Part model, mm, in its own coordinate system. Round coordinates to 2 decimals unless told otherwise and drop trailing zeros. Loops run counter-clockwise (first coordinate to the right, second up) from the corner with the lowest first, then second, coordinate; pieces in that order, holes last. Notation, with made-up numbers: M -10,15 L 48,15 A19 ccw 48,48 Z; hole C 82,-23 d8. An arc over 180 degrees is marked long. Put each result on its own line as item: value. Start each with the question number.
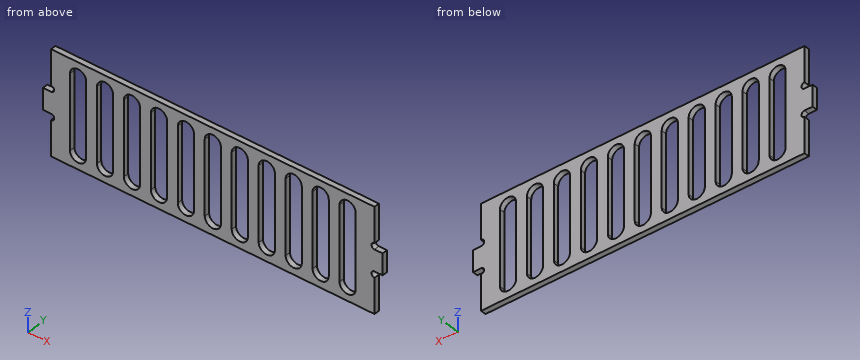
```python
from build123d import *

# Parameters (mm, degrees)
SKETCH_1_W                 = 120
SKETCH_1_H                 = 39
EXTRUDE_1_DEPTH            = 2
SKETCH_2_W                 = 8
SKETCH_2_H                 = 2
EXTRUDE_2_DEPTH            = 3
SKETCH_3_R                 = 1.15
CUT_EXTRUDE_1_DEPTH        = 66.979163378
CUT_EXTRUDE_2_DEPTH        = 66.979163378
PATTERN_LINEAR_1_COUNT     = 6
PATTERN_LINEAR_1_PITCH     = 10
PATTERN_LINEAR_1_COL_COUNT = 6
PATTERN_LINEAR_1_COL_PITCH = 10


with BuildPart() as part:
    # 草图1 → 凸台-拉伸1 (new body)
    with BuildSketch(Plane(origin=(0, 0, 0), x_dir=(1, 0, 0), z_dir=(0, 1, 0))):
        Rectangle(SKETCH_1_W, SKETCH_1_H)
    extrude(amount=EXTRUDE_1_DEPTH)

    # 草图2 → 凸台-拉伸2 (add)
    with BuildSketch(Plane.ZY.offset(60)):
        with Locations((0, 1)):
            Rectangle(SKETCH_2_W, SKETCH_2_H)
    extrude_2 = extrude(amount=EXTRUDE_2_DEPTH)

    # 草图3 → 切除-拉伸1 (cut, through all)
    with BuildSketch(Plane(origin=(0, 2, 0), x_dir=(1, 0, 0), z_dir=(0, 1, 0))):
        with Locations((-60, 5.15)):
            Circle(SKETCH_3_R)
        with Locations((-60, -5.15)):
            Circle(SKETCH_3_R)
    cut_extrude_1 = extrude(amount=-CUT_EXTRUDE_1_DEPTH, mode=Mode.SUBTRACT)

    # 镜向1: 凸台-拉伸2, 切除-拉伸1 across plane
    add(extrude_2.mirror(Plane(origin=(0, 0, 0), x_dir=(0, 0, 1), z_dir=(1, 0, 0))))
    add(cut_extrude_1.mirror(Plane(origin=(0, 0, 0), x_dir=(0, 0, 1), z_dir=(1, 0, 0))), mode=Mode.SUBTRACT)

    # 草图4 → 切除-拉伸2 (cut, through all)
    with BuildSketch(Plane(origin=(0, 2, 0), x_dir=(1, 0, 0), z_dir=(0, 1, 0))):
        with BuildLine():
            ThreePointArc((-3, -14), (0, -11), (3, -14))
            Line((3, -14), (3, 14))
            ThreePointArc((3, 14), (0, 11), (-3, 14))
            Line((-3, 14), (-3, -14))
        make_face()
        with BuildLine():
            ThreePointArc((-3, 14), (0, 11), (3, 14))
            Line((3, 14), (-3, 14))
        make_face()
        with BuildLine():
            Line((-3, 14), (3, 14))
            ThreePointArc((3, 14), (0, 17), (-3, 14))
        make_face()
        with BuildLine():
            ThreePointArc((-3, -14), (0, -17), (3, -14))
            Line((3, -14), (-3, -14))
        make_face()
        with BuildLine():
            Line((-3, -14), (3, -14))
            ThreePointArc((3, -14), (0, -11), (-3, -14))
        make_face()
    cut_extrude_2 = extrude(amount=-CUT_EXTRUDE_2_DEPTH, mode=Mode.SUBTRACT)

    # 阵列(线性)1: 切除-拉伸2 ×6
    with Locations(*[(-i * PATTERN_LINEAR_1_PITCH, 0, 0) for i in range(1, PATTERN_LINEAR_1_COUNT)]):
        add(cut_extrude_2, mode=Mode.SUBTRACT)

    # 阵列(线性)1 col: 切除-拉伸2 ×6
    with Locations(*[(i * PATTERN_LINEAR_1_COL_PITCH, 0, 0) for i in range(1, PATTERN_LINEAR_1_COL_COUNT)]):
        add(cut_extrude_2, mode=Mode.SUBTRACT)


solid = part.part
```
1. Wall check: L1, parallel to Z at x = -30, y = 1.4; L2, parallel to Z at x = 19, y = 0.5. Give the ranges that are in metal, low to high.
2. Cut at A-A, the plane x = -30. Give the cut face in (y, z), and give its area (3 significant figures).
3. Cut at B-B, the plane y = 1.3. Give the number of separate pieces and of enclosed holes in the cut face, and give its area (3 significant figures).
4. Drop flat-ended pins along their axis: pin 1 (1 mm diameter, centred on y = 1, z = 6, fed in from -X); pin 2 (0.6 mm diameter, centred on y = 1, z = 10.5, fed in from +X); pin 3 (2 mm diameter, centred on x = -48.5, z = 6, fed in from -Y); pin 4 (1 mm diameter, centred on x = 61, y = 0.5, fed in from -Z). Give the stop position or say it passes through.
Results list:
1. L1: z = -19.5 to -17, 17 to 19.5
1. L2: z = -19.5 to -16.83, 16.83 to 19.5
2. outline: M 0,-19.5 L 2,-19.5 L 2,-17 L 0,-17 Z; M 0,17 L 2,17 L 2,19.5 L 0,19.5 Z
2. area: 10.0 mm^2
3. separate pieces: 1
3. enclosed holes: 11
3. area: 2,560 mm^2
4. pin 1: stops at x = -60
4. pin 2: stops at x = 60
4. pin 3: passes through
4. pin 4: stops at z = -4
